from build123d import *

# Parameters (mm, degrees)
SKETCH1_R           = 1.5
SKETCH1_W           = 71.428571428
SKETCH1_H           = 3.175
SKETCH1_W_2         = 20
SKETCH1_W_3         = 18.5
BOSS_EXTRUDE1_DEPTH = 3.175


with BuildPart() as part:
    # Sketch1 → Boss-Extrude1 (new body)
    with BuildSketch(Plane.XY):
        Polygon((0, 0), (0, 132.75), (0, 252.75), (328.222222222, 252.75), (363, 252.75), (363, 228.115), (363, 132.75), (357.142857143, 132.75), (357.142857143, 129.575), (428.571428571, 129.575), (428.571428571, 132.75), (550, 132.75), (550, 0), (428.571428571, 0), (428.571428571, 3.175), (357.142857143, 3.175), (357.142857143, 0), (285.714285714, 0), (285.714285714, 3.175), (214.285714286, 3.175), (214.285714286, 0), (142.857142857, 0), (142.857142857, 3.175), (71.428571429, 3.175), (71.428571429, 0), align=None)
        with Locations((56.175, 246.575)):
            Circle(SKETCH1_R, mode=Mode.SUBTRACT)
        with Locations((158.920833333, 135.75)):
            Circle(SKETCH1_R, mode=Mode.SUBTRACT)
        with Locations((158.920833333, 246.575)):
            Circle(SKETCH1_R, mode=Mode.SUBTRACT)
        with Locations((254.079166667, 246.575)):
            Circle(SKETCH1_R, mode=Mode.SUBTRACT)
        with Locations((254.079166667, 135.75)):
            Circle(SKETCH1_R, mode=Mode.SUBTRACT)
        with Locations((356.825, 135.75)):
            Circle(SKETCH1_R, mode=Mode.SUBTRACT)
        with Locations((356.825, 246.575)):
            Circle(SKETCH1_R, mode=Mode.SUBTRACT)
        with Locations((56.175, 135.75)):
            Circle(SKETCH1_R, mode=Mode.SUBTRACT)
        with Locations((107.142857143, 131.1625)):
            Rectangle(SKETCH1_W, SKETCH1_H, mode=Mode.SUBTRACT)
        with Locations((250, 131.1625)):
            Rectangle(SKETCH1_W, SKETCH1_H, mode=Mode.SUBTRACT)
        with Locations((536, 60.0875)):
            Rectangle(SKETCH1_W_2, SKETCH1_H, mode=Mode.SUBTRACT)
        with Locations((536, 72.6625)):
            Rectangle(SKETCH1_W_2, SKETCH1_H, mode=Mode.SUBTRACT)
        with Locations((27.75, 33.2875)):
            Rectangle(SKETCH1_W_3, SKETCH1_H, mode=Mode.SUBTRACT)
        with Locations((27.75, 99.4625)):
            Rectangle(SKETCH1_W_3, SKETCH1_H, mode=Mode.SUBTRACT)
    extrude(amount=BOSS_EXTRUDE1_DEPTH)


solid = part.part
Part model, mm, in its own coordinate system. Give positions to 0.01 mm unless a question says otherwise; leave off trailing zeros. Order: outer loops, then holes, each group sorted by start corner. A loop starts at its lowest first (then second) coordinate and runs counter-clockwise, first axis right, second up. Notation, with made-up numbers: (-15.75, -5.5) - (32.25, -5.5) arc R25 cw to (32.25, 30.5) - close; hole circle Ø8 at (29.5, 74). An arc over 180 degrees is marked (long way). Use a Markdown table: item, result.
1) Flat gauge pins, fed straight in: P1, Ø1.6, axis at x = 540.5, z = 1.5, coming from the +Y side; P2, Ø2.5, axis at x = 56.175, y = 135.75, coming from the -Z side. Where does each tip first touch, or does it go through?
Checked values:
| item | result |
|---|---|
| P1 | y = 132.75 |
| P2 | through |
2) Saw through at D-D on z = 2.5. Count the separate pieces of the cut face and the enclosed holes in it, plus the area to 3 significant figures.
Checked values:
| item | result |
|---|---|
| separate pieces | 1 |
| enclosed holes | 14 |
| area | 115,000 mm² |
3) Saw through at A-A on x = 87. List the corners of the cut face in (y, z) (3 decimals), plus the area to 3 significant figures.
Checked values:
| item | result |
|---|---|
| outline | (3.175, 0) - (129.575, 0) - (129.575, 3.175) - (3.175, 3.175) - close; (132.75, 0) - (252.75, 0) - (252.75, 3.175) - (132.75, 3.175) - close |
| area | 782 mm² |
4) Saw through at C-C on x = 467. List the corners of the cut face in (y, z) (3 decimals).
Checked values:
| item | result |
|---|---|
| outline | (0, 0) - (132.75, 0) - (132.75, 3.175) - (0, 3.175) - close |
5) Probe L1, parallel to X at y = 135.75, z = 2 (3 decimals); L2, parallel to Y at x = 254.5, z = 2.2 (3 decimals); L3, parallel to Y at x = 120, z = 1.1 (3 decimals). List the from-to ranges inside material, lowest first. Write a range as from..to.
Checked values:
| item | result |
|---|---|
| L1 | 0..54.675, 57.675..157.421, 160.421..252.579, 255.579..355.325, 358.325..363 |
| L2 | 3.175..129.575, 132.75..134.31, 137.19..245.135, 248.015..252.75 |
| L3 | 3.175..129.575, 132.75..252.75 |
6) Saw through at B-B on y = 185. List the corners of the cut face in (x, z) (3 decimals), plus the area to 3 significant figures.
Checked values:
| item | result |
|---|---|
| outline | (0, 0) - (363, 0) - (363, 3.175) - (0, 3.175) - close |
| area | 1,150 mm² |
